Source: CAD feature listing. Evaluate the final solid. Frame: model axes, mm. A direction names the side the tool comes from. Round coordinates to 2 decimals unless told otherwise and drop trailing zeros. Loops run counter-clockwise (first coordinate to the right, second up) from the corner with the lowest first, then second, coordinate; pieces in that order, holes last. Notation, with made-up numbers: (-12, 27.5) - (-6, 27.5) arc R35 ccw to (-6, 65.5) - close; hole circle Ø9 at (28.25, 31.25). An arc over 180 degrees is marked (long way). Write item = value, one per line. Start each with the question number.
from build123d import *

# Parameters (mm, degrees)
F0_W     = 20
F0_H     = 5
F1_DEPTH = 200
F2_W     = 30
F2_H     = 10
F3_DEPTH = 5


with BuildPart() as f1:
    # F0 (on Top) → F1 (new body)
    with BuildSketch(Plane.XY):
        Polygon((15, -7.5), (15, 7.5), (-15, 7.5), (-15, -7.5), (-10, -7.5), (-10, -2.5), (10, -2.5), (10, -7.5), align=None)
        with Locations((0, -5)):
            Rectangle(F0_W, F0_H)
        with Locations((0, -10)):
            Rectangle(F0_W, F0_H)
    extrude(amount=F1_DEPTH)

    # F2 (on face) → F3 (join)
    with BuildSketch(Plane(origin=(0, 7.5, 0), x_dir=(-1, 0, 0), z_dir=(0, 1, 0))):
        with Locations((0, 195)):
            Rectangle(F2_W, F2_H)
    extrude(amount=F3_DEPTH)


solid = f1.part
(1) Pin query (flat end, axial travel): P1, Ø4, axis at y = -11, z = 113.5, coming from the -X side; P2, Ø2, axis at y = -9.5, z = 167.5, coming from the +X side; P3, Ø2.5, axis at x = 11.5, z = 100, coming from the -Y side. Return the tip coordinate at first contact, or that it passes through.
(2) Material intervals for line 1 along Y through (x, z) = (13.75, 147); line 2 along Y through (x, z) = (-4.75, 133.5); line 3 along Z through (x, y) = (10.75, 9.5), sorted ascending. Write a range as from..to.
(3) Cut plane D-D (y = -9.5). Output: boundary loops of the cut face in (x, z), and give its area (3 significant figures).
(4) Cut plane A-A (z = 81). Output: boundary loops of the cut face in (x, y).
(5) Cut plane C-C (y = 9.75). Output: boundary loops of the cut face in (x, z), and give its area (3 significant figures).
(6) Cut plane B-B (x = -6.5). Output: boundary loops of the cut face in (y, z).
(7) Access query for faces 1 (the face through (0, 7.5, 94)), 2 (the face through (10, -10, 99)), 3 (the face through (-15, 0, 99)), 4 (the face through (0, -12.5, 99)), 5 (the face through (-13, -7.5, 99)). Directions: +Z, -Z, +X, -X, +Y, -Y. A direction counts if a zero-diameter tool reaches every point of the face in a straight line with its end or side. Return the directions, or none.
Solution:
q1.P1 = -10
q1.P2 = 10
q1.P3 = -7.5
q2.line_1 = -7.5..7.5
q2.line_2 = -12.5..7.5
q2.line_3 = 190..200
q3.outline = (-10, 0) - (10, 0) - (10, 200) - (-10, 200) - close
q3.area = 4,000 mm^2
q4.outline = (-15, -7.5) - (-10, -7.5) - (-10, -12.5) - (10, -12.5) - (10, -7.5) - (15, -7.5) - (15, 7.5) - (-15, 7.5) - close
q5.outline = (-15, 190) - (15, 190) - (15, 200) - (-15, 200) - close
q5.area = 300 mm^2
q6.outline = (-12.5, 0) - (7.5, 0) - (7.5, 190) - (12.5, 190) - (12.5, 200) - (-12.5, 200) - close
q7.face_1 = -Z, +X, -X, +Y
q7.face_2 = +Z, -Z, +X, -Y
q7.face_3 = +Z, -Z, -X, +Y, -Y
q7.face_4 = +Z, -Z, +X, -X, -Y
q7.face_5 = +Z, -Z, -X, -Y
